Here's the drawing with two shaded views (mm, measured from the low corner). I have some questions. Round coordinates to 2 decimals unless told otherwise and drop trailing zeros. Loops run counter-clockwise (first coordinate to the right, second up) from the corner with the lowest first, then second, coordinate; pieces in that order, holes last.
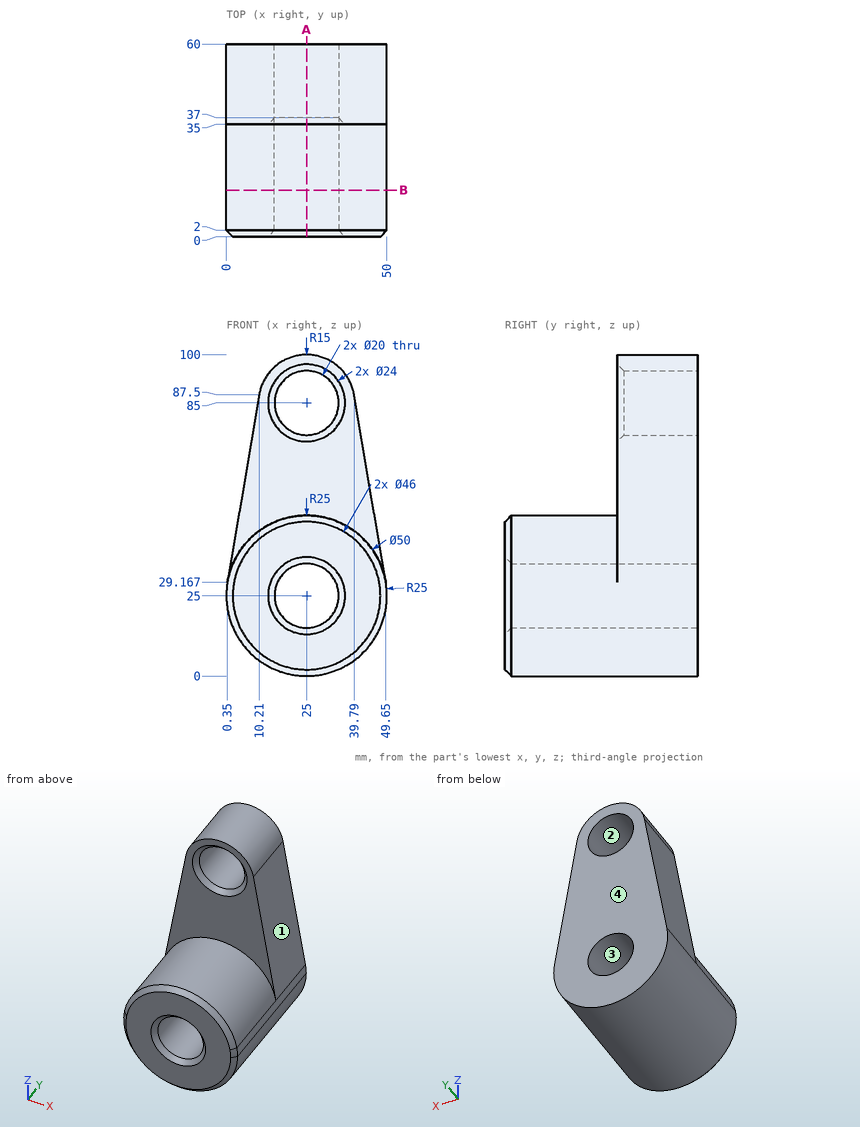
Item 1: If we section it at B-B, the plane y = 14.5: Please give me the cut outline in (x, z).
Results list:
outline: (49.65, 29.17) arc R25 ccw (long way) to (50, 25) arc R25 ccw to start; hole circle Ø20 at (25, 25)
Item 2: We'd pull the mould along Z, two halves only. Please class the marked faces 1, 2, 3 and 4: released by +Z, released by -Z, zero draft, split by the parting line, or undercut.
Results list:
face 1: released by +Z
face 2: undercut
face 3: undercut
face 4: zero draft
Item 3: If we section it at A-A, the plane x = 25: Please give me the cut outline in (y, z), then the cut area to 3 significant figures.
Results list:
outline: (0, 2) - (2, 0) - (60, 0) - (60, 15) - (2, 15) - (0, 13) - close; (0, 37) - (2, 35) - (60, 35) - (60, 75) - (37, 75) - (35, 73) - (35, 50) - (2, 50) - (0, 48) - close; (35, 97) - (37, 95) - (60, 95) - (60, 100) - (35, 100) - close
area: 2,540 mm2
Item 4: Will these pins go through, and if not, where does the flat tip stop? pin 1 (2 mm diameter, centred on x = 22.5, y = 14, fed in from -Z) (3 decimals); pin 2 (5 mm diameter, centred on y = 49.5, z = 80, fed in from -X); pin 3 (6 mm diameter, centred on x = 34, y = 52.5, fed in from -Z).
Results list:
pin 1: stops at z = 0.045
pin 2: stops at x = 8.52
pin 3: stops at z = 0.73
Item 5: If I drill on line 1 along Z through (x, y) = (25, 46); line 2 along Z through (x, y) = (31.5, 34.5); line 3 along Y through (x, z) = (18.5, 51), over which ranges is the centre line in solid material (lowest first)?
Results list:
line 1: z = 0 to 15, 35 to 75, 95 to 100
line 2: z = 0.86 to 17.4, 32.6 to 49.14
line 3: y = 35 to 60
